Source: CAD feature listing. Evaluate the final solid. Frame: model axes, mm. Round coordinates to 2 decimals unless told otherwise and drop trailing zeros. Order: outer loops, then holes, each group sorted by start corner. A loop starts at its lowest first (then second) coordinate and runs counter-clockwise, first axis right, second up. Notation, with made-up numbers: (-25, 86) -> (27, 86) arc R32 cw to (27, 117) -> close; hole circle Ø1 at (37, -1.75). An arc over 180 degrees is marked (long way). Use a Markdown table: item, result. Add a question column.
```python
from build123d import *

# Parameters (mm, degrees)
SKETCH_1_R             = 2
SM_BASE_FLANGE_1_DEPTH = 3


# Sheet-metal steps are written as plain solids
with BuildPart() as part:
    # Sketch 1 → Базовая кромка1 (new body)
    with BuildSketch(Plane(origin=(0, 0, 0), x_dir=(0, 0, -1), z_dir=(1, 0, 0))):
        with BuildLine():
            Line((-49.62399479, 0), (0, 0))
            Line((0, 0), (0, 200))
            Line((0, 200), (-190, 200))
            Line((-190, 200), (-190, 141))
            ThreePointArc((-190, 141), (-109.877663421, 80.390369629), (-49.62399479, 0))
        make_face()
        with Locations((-185, 192)):
            Circle(SKETCH_1_R, mode=Mode.SUBTRACT)
        with Locations((-165, 192)):
            Circle(SKETCH_1_R, mode=Mode.SUBTRACT)
        with Locations((-25, 192)):
            Circle(SKETCH_1_R, mode=Mode.SUBTRACT)
        with Locations((-5, 192)):
            Circle(SKETCH_1_R, mode=Mode.SUBTRACT)
    extrude(amount=-SM_BASE_FLANGE_1_DEPTH)


solid = part.part
```
1) Section A-A on x = -0.6. Output: boundary loops of the cut face in (y, z), then the cut area to 3 significant figures.
2) Draft query along X for faces 1 (the flat face through (0, 124, 75)), 2 (the flat face through (-3, 124, 75)), 3 (the cylindrical face through (-1.479, 81.388, 110.875)). Return one class per face: pulls with the +X half, pulls with the -X half, needs draft (parallel to the pull), parting line crosses it, or undercut.
3) Line query: probe 1 along Z at (x, y) = (-2.05, 192); probe 2 along Y at (x, z) = (-1.6, 5); probe 3 along Y at (x, z) = (-0.7, 185). Output: solid intervals per line, ascending. Write a range as from..to.
4) Section C-C on z = 113. Output: boundary loops of the cut face in (x, y), then the cut area to 3 significant figures.
5) First-contact query: pin 1 Ø6.5 at (y, z) = (192, 165) entering from +X. Flat tip, straight axial feed; report the tip coordinate or a pass-through.
6) Section B-B on y = 128. Output: boundary loops of the cut face in (x, z).
Conclusion:
| question | item | result |
|---|---|---|
| 1 | outline | (0, 0) -> (200, 0) -> (200, 190) -> (141, 190) arc R360 cw to (0, 49.62) -> close; hole circle Ø4 at (192, 5); hole circle Ø4 at (192, 25); hole circle Ø4 at (192, 165); hole circle Ø4 at (192, 185) |
| 1 | area | 26,200 mm^2 |
| 2 | face 1 | pulls with the +X half |
| 2 | face 2 | pulls with the -X half |
| 2 | face 3 | needs draft |
| 3 | probe 1 | z = 0..3, 7..23, 27..163, 167..183, 187..190 |
| 3 | probe 2 | y = 0..190, 194..200 |
| 3 | probe 3 | y = 138.17..190, 194..200 |
| 4 | outline | (-3, 83.49) -> (0, 83.49) -> (0, 200) -> (-3, 200) -> close |
| 4 | area | 350 mm^2 |
| 5 | pin 1 | stops at x = 0 |
| 6 | outline | (-3, 0) -> (0, 0) -> (0, 168.44) -> (-3, 168.44) -> close |
